Design review of the part built by this model. Coordinates are the model's own, in mm. A direction names the side the tool comes from. Coordinates: 2 decimals unless noted, no trailing zeros. Loops run counter-clockwise (first coordinate to the right, second up) from the corner with the lowest first, then second, coordinate; pieces in that order, holes last. Notation, with made-up numbers: M 8,24 L 17,24 A28 cw 17,48 Z; hole C -19,20 d8. An arc over 180 degrees is marked long. Write item = value, one per line. Start each with the question number.
Autodesk Fusion 360 part; units mm, degrees
sketch "Sketch1" plane through (0, 0, 0) normal (0, 0, 1) x (1, 0, 0)
  circle A0 centre (0, 0) radius 75
  dimension "d1" = 150
extrude "Extrude1" add sketch "Sketch1" along normal blind 10 makes body 1
sketch "Sketch2" plane through (0, 0, 10) normal (0, 0, 1) x (-1, 0, 0)
  circle A0 centre (0, 0) radius 75
sketch "Sketch3" plane through (0, 0, 10) normal (0, 0, 1) x (-1, 0, 0)
  circle A0 centre (0, 0) radius 37.5
  dimension "d4" = 75
extrude "Extrude2" add sketch "Sketch3" along normal blind 200 bodies 1
sketch "Sketch4" plane through (0, 0, 10) normal (0, 0, 1) x (-1, 0, 0)
  circle A0 centre (0, 0) radius 37.5
  line L0 (60.6763, 44.0839) -> (28.3156, 20.5725)
  line L1 (-23.1763, 71.3292) -> (-10.8156, 33.287)
  line L2 (-75, 0) -> (-35, 0)
  line L3 (-23.1763, -71.3292) -> (-10.8156, -33.287)
  line L4 (60.6763, -44.0839) -> (28.3156, -20.5725)
  line L5 (75, 0) -> (55, 0)
  line L6 (75, 0) -> (55, 0)
  line L7 (23.1763, 71.3292) -> (16.9959, 52.3081)
  line L8 (-60.6763, 44.0839) -> (-44.4959, 32.3282)
  line L9 (-60.6763, -44.0839) -> (-44.4959, -32.3282)
  line L10 (23.1763, -71.3292) -> (16.9959, -52.3081)
  line L11 (-10.8156, 33.287) -> (-23.1763, 71.3292)
  line L12 (-23.1763, 71.3292) -> (-26.0294, 70.4022)
  line L13 (-26.0294, 70.4022) -> (-13.6688, 32.3599)
  line L14 (-13.6688, 32.3599) -> (-10.8156, 33.287)
  line L15 (-75, 0) -> (-75, -3)
  line L16 (-35, -3) -> (-35, 0)
  line L17 (-75, -3) -> (-35, -3)
  line L18 (-23.1763, -71.3292) -> (-20.3231, -72.2563)
  line L19 (-7.9624, -34.214) -> (-10.8156, -33.287)
  line L20 (-20.3231, -72.2563) -> (-7.9624, -34.214)
  line L21 (60.6763, -44.0839) -> (62.4396, -41.6568)
  line L22 (30.079, -18.1454) -> (28.3156, -20.5725)
  line L23 (62.4396, -41.6568) -> (30.079, -18.1454)
  line L24 (60.6763, 44.0839) -> (58.9129, 46.5109)
  line L25 (26.5522, 22.9995) -> (28.3156, 20.5725)
  line L26 (58.9129, 46.5109) -> (26.5522, 22.9995)
  point P0 (75, 0)
  dimension "d9" = 20
  dimension "d11" = 360
  dimension "d12" = 3
  dimension "d14" = 360
extrude "Extrude3" add sketch "Sketch4" along normal blind 35 separate body contours A0 L0 L25 L26 | A0 L0 L24 L26 | A0 L4 L21 L23 | A0 L4 L22 L23 | A0 L1 L11 L13 L14 | A0 L1 L11 L12 L13 | A0 L3 L18 L20 | A0 L3 L19 L20 | A0 L2 L16 L17 | A0 L2 L15 L17 makes body 2 at (16.2029, 59.5755, 21.6667) makes body 3 at (19.056, -58.6485, 33.3333) makes body 4 at (-48.126, -38.6738, 33.3333) makes body 5 at (61.6667, 3, 33.3333) makes body 6 at (-49.8894, 36.2468, 33.3333)
sketch "Sketch5" plane through (0, 0, 10) normal (0, 0, 1) x (-1, 0, 0)
  line L0 (75, 3) -> (55, 3)
  line L1 (20.3231, 72.2563) -> (14.1428, 53.2352)
  line L2 (-62.4396, 41.6568) -> (-46.2593, 29.9011)
  line L3 (-58.9129, -46.5109) -> (-42.7326, -34.7552)
  line L4 (26.0294, -70.4022) -> (19.8491, -51.3811)
  point P0 (62.4396, -41.6568)
  point P1 (30.079, -18.1454)
  dimension "d19" = 20
  dimension "d21" = 360
hole "Hole1" at (-55, -3, 10) at (-14.1428, -53.2352, 10) at (-19.8491, 51.3811, 10) at (42.7326, 34.7552, 10) at (46.2593, -29.9011, 10) direction (0, 0, -1) diameter 12.023 depth 10 tip angle 118 counterbore diameter 18 counterbore depth 1 bodies 1
fillet "Fillet1" radius 5 1 edges at (34.9623, -13.5606, 10) on bodies 1
combine "Combine1" operation add target body 1 tool bodies 4 3 5 6 2
chamfer "Chamfer1" distance 35 distance2 35 5 edges at (75, 1.5, 45) (21.7497, 71.7928, 45) (-61.558, 42.8704, 45) (24.6029, -70.8657, 45) (-59.7946, -45.2974, 45) measured on face at (62.4955, 1.3337, 45) measured on face at (18.0438, 59.8489, 45) measured on face at (-51.3439, 35.655, 45) measured on face at (20.5806, -59.0247, 45) measured on face at (-49.7761, -37.8129, 45) on bodies 1
sketch "Sketch6" plane through (0, 0, 210) normal (0, 0, 1) x (-1, 0, 0)
  circle A0 centre (0, 0) radius 37.5
  line L0 (-21.209, 21.209) -> (21.209, 21.209)
  line L1 (21.209, 21.209) -> (21.209, -21.209)
  line L2 (21.209, -21.209) -> (-21.209, -21.209)
  line L3 (-21.209, -21.209) -> (-21.209, 21.209)
  line L4 (-21.209, 21.209) -> (21.209, -21.209) construction
  line L5 (21.209, 21.209) -> (-21.209, -21.209) construction
  dimension "d31" = 42.418
  dimension "d32" = 42.418
extrude "Extrude9" cut 1 faces at (-9.3028, -10.3652, 210) along direction (0, 0, -1) blind 20 on bodies 1 bodies 1
sketch "Sketch22" plane through (0, 0, 190) normal (0, 0, 1) x (-1, 0, 0)
  circle A0 centre (0, 0) radius 37.5
sketch "Sketch23" plane through (0, 0, 190) normal (0, 0, 1) x (-1, 0, 0)
  line L0 (-21.2, -21.2) -> (21.2, -21.2)
  line L1 (21.2, -21.2) -> (21.2, 21.2)
  line L2 (21.2, 21.2) -> (-21.2, 21.2)
  line L3 (-21.2, 21.2) -> (-21.2, -21.2)
  line L4 (-21.2, -21.2) -> (21.2, 21.2) construction
  line L5 (21.2, -21.2) -> (-21.2, 21.2) construction
  dimension "d103" = 42.4
  dimension "d104" = 42.4
extrude "Extrude10" cut sketch "Sketch23" against normal blind 48.006 bodies 1
sketch "Sketch24" plane through (0, 0, 190) normal (0, 0, 1) x (-1, 0, 0)
  line L0 (21.2, -21.2) -> (21.2, -21.962)
  line L1 (-21.2, -21.2) -> (-21.2, -21.962)
  line L2 (21.2, -21.2) -> (-21.2, -21.2)
  line L3 (-21.2, -21.962) -> (21.2, -21.962)
  point P0 (21.2, -21.2)
  point P1 (-21.2, -21.2)
  dimension "d107" = 0.762
  dimension "d108" = 0.762
extrude "Extrude11" cut sketch "Sketch24" against normal blind 48.006 bodies 1
sketch "Sketch26" plane through (0, 21.962, 0) normal (0, -1, 0) x (1, 0, 0)
  line L0 (21.2, 190) -> (-21.2, 190)
  line L1 (-21.2, 190) -> (-21.2, 141.994)
  line L2 (-21.2, 141.994) -> (21.2, 141.994)
  line L3 (21.2, 141.994) -> (21.2, 190)
  line L4 (0, 141.994) -> (0, 142.248)
  line L5 (0, 142.248) -> (5.715, 142.248)
  line L6 (0, 142.248) -> (-5.715, 142.248)
  line L7 (5.715, 142.248) -> (5.715, 151.341)
  line L8 (-5.715, 142.248) -> (-5.715, 151.341)
  line L9 (-5.715, 151.341) -> (5.715, 151.341)
  dimension "d111" = 0.254
  dimension "d112" = 5.715
  dimension "d113" = 5.715
  dimension "d114" = 9.093
  dimension "d115" = 9.093
extrude "Extrude12" cut sketch "Sketch26" against normal blind 55 contours L5 L6 L7 L8 L9 bodies 1
sketch "Sketch27" plane through (0, 0, 190) normal (0, 0, 1) x (-1, 0, 0)
  circle A0 centre (0, 0) radius 37.5
  line L0 (-0.1682, -37.4996) -> (-0.1233, -27.4997)
  line L1 (37.4996, -0.1682) -> (27.4997, -0.1233)
  line L2 (0.1682, 37.4996) -> (0.1233, 27.4997)
  line L3 (-37.4996, 0.1682) -> (-27.4997, 0.1233)
  dimension "d118" = 10
  dimension "d120" = 360
hole "Hole5" at (27.4997, -0.1233, 190) at (-0.1233, -27.4997, 190) at (0.1233, 27.4997, 190) at (-27.4997, 0.1233, 190) direction (0, 0, -1) diameter 3.332 depth 35 tip angle 118 bodies 1
(1) Tool access review of faces 1 (the flat face through (16.176, -49.784, 23.366)), 2 (the flat face through (45, -42, 10)), 3 (the flat face through (-44.053, 28.298, 23.366)): name each direction out of +Z, -Z, +X, -X, +Y, -Y from which nothing blocks a thin tool from reaching the whole face with its end or side.
(2) Take a section at D-D (z = 168). State the section outline as (x, y) points.
(3) Mouldability with a two-part tool opening along X and no side actions: class faces 4 (the flat face through (16.176, 49.784, 23.366)), 5 (the flat face through (-47.589, 32.747, 27.259)), 6 (the cylindrical face through (46.391, 39.526, 4.437)) as +X half, -X half, draft (parallel to the pull), parting line (faces both ways), or undercut.
(4) Take a section at C-C (z = 34.5). State the section outline as (x, y) points, plus the area to 3 significant figures.
(5) To check wall thickness, follow L1, parallel to X at y = 23.5, z = 80; L2, parallel to Z at x = -35, y = -34; L3, parallel to Y at x = -55, z = 3.5. State the ranges of each line that lie inside material, in increasing order.
(6) Take a section at B-B (x = -55). State the section outline as (y, z) points.
(7) Take a section at A-A (y = 52). State the section outline as (x, z) points, plus the area to 3 significant figures.
(8) Insertion check: pin 1 (21.5 mm diameter, centred on y = -2.5, z = 176, fed in from -X); pin 2 (2 mm diameter, centred on x = -11, z = 135, fed in from -Y); pin 3 (3 mm diameter, centred on x = -31, y = -23, fed in from +Z); pin 4 (2.5 mm diameter, centred on y = 30.5, z = 145, fed in from +X). Each pin has a flat end and moves straight along its axis. Give the tip position at first contact, or say it passes through.
Results list:
q1.face_1 = +Z, -Y
q1.face_2 = +Z, +X
q1.face_3 = +Z, -X
q2.outline = C 0,0 d75; hole C -27.5,0.12 d3.33; hole M -21.2,-21.2 L 21.2,-21.2 L 21.2,21.96 L -21.2,21.96 Z; hole C -0.12,-27.5 d3.33; hole C 0.12,27.5 d3.33; hole C 27.5,-0.12 d3.33
q3.face_4 = +X half
q3.face_5 = -X half
q3.face_6 = undercut
q4.outline = M -42.62,27.26 L -32,19.54 A37.5 ccw -30.34,-22.04 L -40.86,-29.69 L -39.1,-32.11 L -28.48,-24.4 A37.5 ccw 11.59,-35.66 L 15.61,-48.03 L 18.46,-47.11 L 14.4,-34.62 A37.5 ccw 37.5,0 L 50.51,0 L 50.51,3 L 37.38,3 A37.5 ccw 11.59,35.66 L 15.61,48.03 L 12.75,48.96 L 8.7,36.48 A37.5 ccw -30.34,22.04 L -40.86,29.69 Z
q4.area = 4,610 mm^2
q5.L1 = -29.22 to 29.22
q5.L2 = 0 to 10
q5.L3 = -50.99 to -9.01, 3.01 to 50.99
q6.outline = M -50.99,0 L -9.01,0 L -9.01,9 L -12,9 L -12,10 L -39.96,10 L -39.96,17.02 L -43.67,14.84 L -43.67,10 L -50.99,10 Z; M 3.01,0 L 50.99,0 L 50.99,10 L 39.96,10 L 39.96,17.02 L 36.25,19.2 L 36.25,10 L 6,10 L 6,9 L 3.01,9 Z
q7.outline = M -54.05,0 L -25.83,0 L -25.83,9 L -28.83,9 L -28.83,10 L -54.05,10 Z; M -13.87,0 L 54.05,0 L 54.05,10 L 16.9,10 L 16.9,30.33 L 13.74,31.31 L 13.74,10 L -10.87,10 L -10.87,9 L -13.87,9 Z
q7.area = 1,020 mm^2
q8.pin_1 = -37.5
q8.pin_2 = -36.14
q8.pin_3 = 190
q8.pin_4 = 23.47
